Work out the finished part from the listing and answer in its coordinate system (mm). A direction names the side the tool comes from. Give positions to 0.01 mm unless a question says otherwise; leave off trailing zeros. Order: outer loops, then holes, each group sorted by start corner. A loop starts at its lowest first (then second) coordinate and runs counter-clockwise, first axis right, second up. Notation, with made-up numbers: M -21.5,75.25 L 23.5,75.25 A17 ccw 23.5,88.25 Z; hole C 7,-12.5 d5. An arc over 180 degrees is marked long. One line per item, written item: value.
from build123d import *

# Parameters (mm, degrees)
BOSS_EXTRU_1_DEPTH = 4


with BuildPart() as part:
    # Esquisse1 → Boss.-Extru.1 (new body)
    with BuildSketch(Plane.XY):
        Polygon((-72.387865901, -137.132902491), (-69.559438777, -134.304475366), (-69.559438777, 89.31574626), (-72.384288507, 92.14774626), (-54.684288507, 109.803057076), (-51.859438777, 106.971057076), (-34.159438777, 124.626367892), (-34.159438777, -169.704475366), (-51.837108306, -152.026805837), (-54.665535431, -154.855232961), (-36.987865901, -172.532902491), (-431.331011652, -172.532902491), (-413.653342122, -154.855232961), (-416.481769247, -152.026805837), (-434.159438777, -169.704475366), (-434.159438777, 124.638670384), (-416.459438777, 106.983359568), (-413.634589046, 109.815359568), (-395.934589046, 92.160048753), (-398.759438777, 89.328048753), (-398.759438777, -134.304475366), (-395.931011652, -137.132902491), align=None)
    extrude(amount=BOSS_EXTRU_1_DEPTH)


solid = part.part
(1) Section A-A, the plane y = -13 is taken. Give the vertices of the cut face in (x, z), then the cut area to 3 significant figures.
Findings:
outline: M -434.16,0 L -398.76,0 L -398.76,4 L -434.16,4 Z; M -69.56,0 L -34.16,0 L -34.16,4 L -69.56,4 Z
area: 283 mm^2
(2) Section B-B, the plane z = 1.5 is taken. Give the vertices of the cut face in (x, y), then the cut area to 3 significant figures.
Findings:
outline: M -434.16,-169.7 L -416.48,-152.03 L -413.65,-154.86 L -431.33,-172.53 L -36.99,-172.53 L -54.67,-154.86 L -51.84,-152.03 L -34.16,-169.7 L -34.16,124.63 L -51.86,106.97 L -54.68,109.8 L -72.38,92.15 L -69.56,89.32 L -69.56,-134.3 L -72.39,-137.13 L -395.93,-137.13 L -398.76,-134.3 L -398.76,89.33 L -395.93,92.16 L -413.63,109.82 L -416.46,106.98 L -434.16,124.64 Z
area: 31,400 mm^2
(3) Section C-C, the plane x = -218 is taken. Give the vertices of the cut face in (y, z).
Findings:
outline: M -172.53,0 L -137.13,0 L -137.13,4 L -172.53,4 Z
(4) Find the intervals of material crossed by probe 1 along X at (y, z) = (-114, 1.8); probe 2 along Y at (x, z) = (-93.5, 1.75); probe 3 along X at (y, z) = (94.5, 3.7), in increasing order. Write a range as from..to.
Findings:
probe 1: x = -434.16..-398.76, -69.56..-34.16
probe 2: y = -172.53..-137.13
probe 3: x = -434.16..-398.28, -70.03..-34.16
(5) Section D-D, the plane x = -63 is taken. Give the vertices of the cut face in (y, z).
Findings:
outline: M -172.53,0 L 101.51,0 L 101.51,4 L -172.53,4 Z
(6) Determine the mould class of faces 4 (the flat face through (-422.6, -163.8, 2)), 5 (the flat face through (-218, -144, 0)), 6 (the flat face through (-425.4, 115.9, 2)) for opening direction X: pulls with the +X half, pulls with the -X half, needs draft (parallel to the pull), parting line crosses it, or undercut.
Findings:
face 4: undercut
face 5: needs draft
face 6: undercut
(7) Which of the six approach directions +Z, -Z, +X, -X, +Y, -Y give full straight-line access (tool end or side, diameter ignored) to faces 1 (the flat face through (-218, -144, 4)), 2 (the flat face through (-63.66, 100.85, 1.97)), 3 (the flat face through (-425.197, -160.742, 1.972))?
Findings:
face 1: +Z, +X, -X, +Y, -Y
face 2: +Z, -Z, +Y
face 3: +Z, -Z
